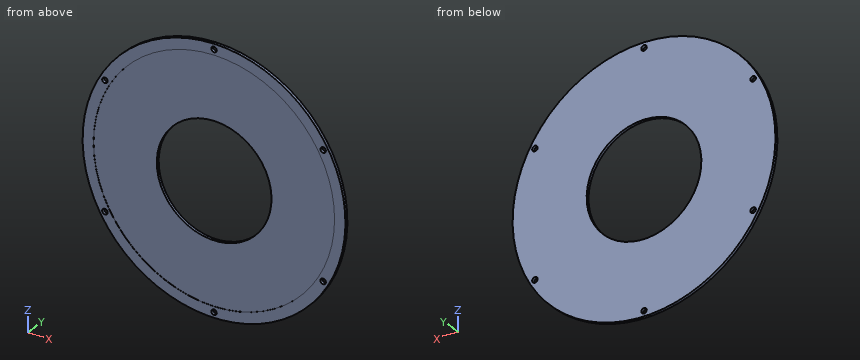
```python
from build123d import *

# Parameters (mm, degrees)
SKETCH1_R           = 70.8759
SKETCH1_R_2         = 1.4732
SKETCH1_R_3         = 65
SKETCH1_R_4         = 57
SKETCH1_R_5         = 30.925
BOSS_EXTRUDE1_DEPTH = 1.6
SKETCH1_3_R         = 65
SKETCH1_3_R_2       = 57
SKETCH1_3_R_3       = 30.925
CUT_EXTRUDE1_DEPTH  = 0.1


with BuildPart() as part:
    # Sketch1 → Boss-Extrude1 (new body)
    # profile 1 of 3: a face of its own
    with BuildSketch(Plane(origin=(0, 0, 0), x_dir=(1, 0, 0), z_dir=(0, 1, 0))):
        with Locations(Location((0, 0, 0), (0, 0, 270))):
            Circle(SKETCH1_R)
        with Locations(Location((0, 67.93795, 0), (0, 0, 270))):
            Circle(SKETCH1_R_2, mode=Mode.SUBTRACT)
        with Locations(Location((58.835990581, 33.968975, 0), (0, 0, 270))):
            Circle(SKETCH1_R_2, mode=Mode.SUBTRACT)
        with Locations(Location((58.835990581, -33.968975, 0), (0, 0, 270))):
            Circle(SKETCH1_R_2, mode=Mode.SUBTRACT)
        with Locations(Location((0, -67.93795, 0), (0, 0, 270))):
            Circle(SKETCH1_R_2, mode=Mode.SUBTRACT)
        with Locations(Location((-58.835990581, -33.968975, 0), (0, 0, 270))):
            Circle(SKETCH1_R_2, mode=Mode.SUBTRACT)
        with Locations(Location((-58.835990581, 33.968975, 0), (0, 0, 270))):
            Circle(SKETCH1_R_2, mode=Mode.SUBTRACT)
        Circle(SKETCH1_R_3, mode=Mode.SUBTRACT)
    # profile 2 of 3: a face of its own
    with BuildSketch(Plane(origin=(0, 0, 0), x_dir=(1, 0, 0), z_dir=(0, 1, 0))):
        Circle(SKETCH1_R_3)
        Circle(SKETCH1_R_4, mode=Mode.SUBTRACT)
    # profile 3 of 3: a face of its own
    with BuildSketch(Plane(origin=(0, 0, 0), x_dir=(1, 0, 0), z_dir=(0, 1, 0))):
        Circle(SKETCH1_R_4)
        with Locations(Location((0, 0, 0), (0, 0, 270))):
            Circle(SKETCH1_R_5, mode=Mode.SUBTRACT)
    extrude(amount=BOSS_EXTRUDE1_DEPTH)

    # Sketch1_3 → Cut-Extrude1 (cut)
    # profile 1 of 2: a face of its own
    with BuildSketch(Plane(origin=(0, 0, 0), x_dir=(1, 0, 0), z_dir=(0, 1, 0))):
        with Locations(Location((0, 0, 0), (0, 0, 270))):
            Circle(SKETCH1_3_R)
        Circle(SKETCH1_3_R_2, mode=Mode.SUBTRACT)
    # profile 2 of 2: a face of its own
    with BuildSketch(Plane(origin=(0, 0, 0), x_dir=(1, 0, 0), z_dir=(0, 1, 0))):
        Circle(SKETCH1_3_R_2)
        with Locations(Location((0, 0, 0), (0, 0, 270))):
            Circle(SKETCH1_3_R_3, mode=Mode.SUBTRACT)
    extrude(amount=CUT_EXTRUDE1_DEPTH, mode=Mode.SUBTRACT)


solid = part.part
```
Input: part model. Units: mm. Frame: model coordinates. Round coordinates to 2 decimals unless told otherwise and drop trailing zeros. Loops run counter-clockwise (first coordinate to the right, second up) from the corner with the lowest first, then second, coordinate; pieces in that order, holes last. Notation, with made-up numbers: M -39.75,-26.75 L 8.25,-26.75 A32 ccw 8.25,10.25 Z; hole C -36.75,-18 d5. An arc over 180 degrees is marked long. Answer in a Markdown table with one row per item. Add a question column.
1. Ray query, probe 1 along X at (y, z) = (0.65, 0) (3 decimals); probe 2 along X at (y, z) = (1.2, 34); probe 3 along Y at (x, z) = (-43.5, 2). Return the intervals inside material, ascending.
2. Section C-C (x = 43). Output: boundary loops of the cut face in (y, z).
3. Section D-D (y = 0.95). Output: boundary loops of the cut face in (x, z) (3 decimals).
4. Section B-B (x = 23). Output: boundary loops of the cut face in (y, z), and give its area (3 significant figures).
5. Section A-A (z = 0). Output: boundary loops of the cut face in (x, y) (3 decimals).
6. Contact query for flat-ended pins moving along their axis: pin 1 (4.5 mm diameter, centred on x = -58.84, z = 33.97, fed in from -Y); pin 2 (1 mm diameter, centred on x = 55, z = -11, fed in from -Y). Output: stop coordinate, or through.
Values follow:
| question | item | result |
|---|---|---|
| 1 | probe 1 | -70.876 to -30.925, 30.925 to 70.876 |
| 1 | probe 2 | -62.19 to -60.31, -57.36 to 57.36, 60.31 to 62.19 |
| 1 | probe 3 | 0.1 to 1.6 |
| 2 | outline | M 0,-56.34 L 1.6,-56.34 L 1.6,56.34 L 0,56.34 L 0,48.74 L 0.1,48.74 L 0.1,-48.74 L 0,-48.74 Z |
| 3 | outline | C 0,0 d141.752; hole C -58.836,-33.969 d2.946; hole C -58.836,33.969 d2.946; hole C 0,0 d61.85; hole C 0,-67.938 d2.946; hole C 0,67.938 d2.946; hole C 58.836,-33.969 d2.946; hole C 58.836,33.969 d2.946 |
| 4 | outline | M 0,-67.04 L 1.6,-67.04 L 1.6,-20.67 L 0.1,-20.67 L 0.1,-60.79 L 0,-60.79 Z; M 0,60.79 L 0.1,60.79 L 0.1,20.67 L 1.6,20.67 L 1.6,67.04 L 0,67.04 Z |
| 4 | area | 140 mm^2 |
| 5 | outline | M -70.876,0 L -65,0 L -65,0.1 L -30.925,0.1 L -30.925,1.6 L -70.876,1.6 Z; M 30.925,0.1 L 65,0.1 L 65,0 L 70.876,0 L 70.876,1.6 L 30.925,1.6 Z |
| 6 | pin 1 | y = 0 |
| 6 | pin 2 | y = 0.1 |
